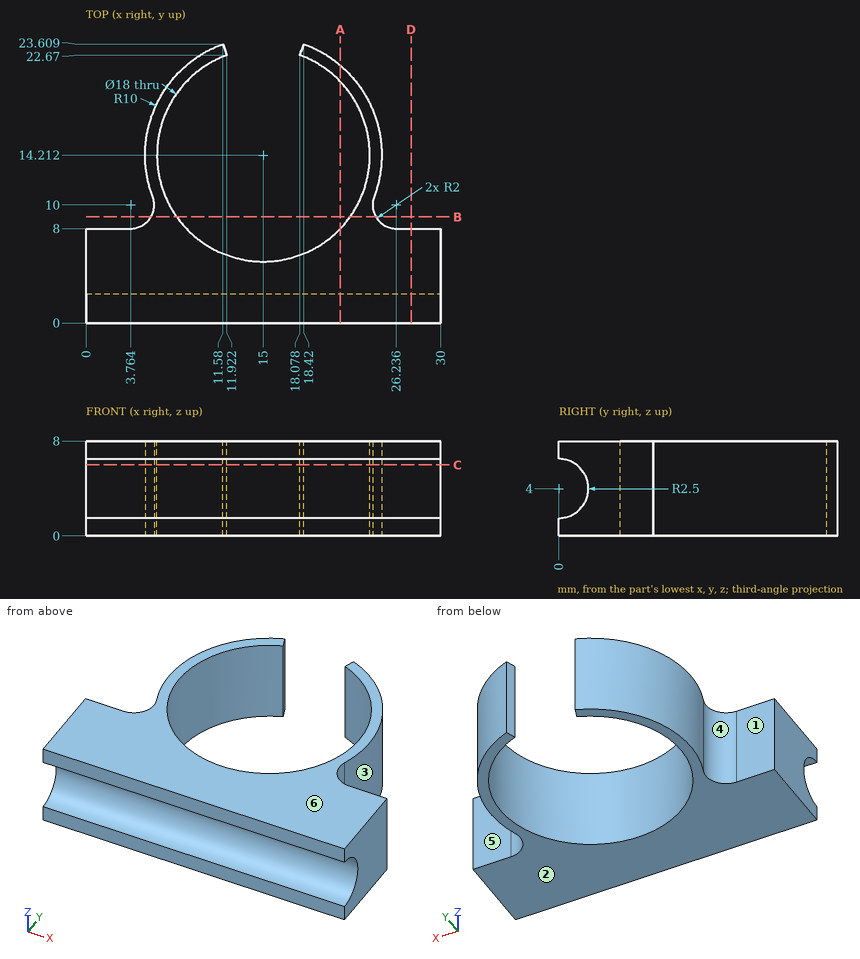
The drawing under review shows one solid part. Ordinate dimensions are in mm from its lowest x, y, z. A direction names the side the tool comes from. Round coordinates to 2 decimals unless told otherwise and drop trailing zeros. Loops run counter-clockwise (first coordinate to the right, second up) from the corner with the lowest first, then second, coordinate; pieces in that order, holes last.
Item 1: For the marked faces 1 and 2, list the 3-axis set-ups (+Z, -Z, +X, -X, +Y, -Y) from which the entire face can be reached by the end or side of a thin tool; tool diameter is ignored.
Determined:
face 1: +Z, -Z, -X, +Y
face 2: -Z, +X, -X, +Y, -Y
Item 2: Clearance check with flat-ended pins moving along their axes: pin 1 Ø4 at (y, z) = (16.5, 6.5) entering from +X; pin 2 Ø3 at (x, y) = (24.5, 16.5) entering from -Z; pin 3 Ø3 at (x, z) = (27.5, 3.5) entering from +Y; pin 4 Ø10 at (x, y) = (14, 12) entering from -Z. State where each tip first meets the part, or that it passes through.
Determined:
pin 1: stops at x = 25
pin 2: stops at z = 0
pin 3: stops at y = 8.01
pin 4: passes through
Item 3: For line 1 (X direction, y = 7.75, z = 3.25) (1 decimal); line 2 (X direction, y = 12, z = 3.25) (1 decimal); line 3 (Y direction, x = 10.75, z = 3.75) (1 decimal), list the stretches that pass through material, from the lowest coordinate up.
Determined:
line 1: x = 0 to 8.7, 21.3 to 30
line 2: x = 5.2 to 6.3, 23.7 to 24.8
line 3: y = 2.5 to 6.3, 22.1 to 23.3
Item 4: Take a section at D-D (x = 27.5). Write out the cut boundary in (y, z).
Determined:
outline: (0, 0) - (8, 0) - (8, 8) - (0, 8) - (0, 6.5) arc R2.5 cw to (0, 1.5) - close
Item 5: Take a section at B-B (y = 9). Write out the cut boundary in (x, z) (1 decimal).
Determined:
outline: (5.5, 0) - (7.7, 0) - (7.7, 8) - (5.5, 8) - close; (22.3, 0) - (24.5, 0) - (24.5, 8) - (22.3, 8) - close
Item 6: Take a section at A-A (x = 21.5). Write out the cut boundary in (y, z).
Determined:
outline: (0, 0) - (7.99, 0) - (7.99, 8) - (0, 8) - (0, 6.5) arc R2.5 cw to (0, 1.5) - close; (20.44, 0) - (21.81, 0) - (21.81, 8) - (20.44, 8) - close
Item 7: Mouldability with a two-part tool opening along Y and no side actions: class the marked faces 3, 4, 5 and 6 as released by +Y, released by -Y, zero draft, split by the parting line, or undercut.
Determined:
face 3: undercut
face 4: undercut
face 5: released by +Y
face 6: zero draft
Item 8: Take a section at C-C (z = 6). Write out the cut boundary in (x, y).
Determined:
outline: (0, 1.5) - (30, 1.5) - (30, 8) - (26.24, 8) arc R2 cw to (24.36, 10.7) arc R10 ccw to (18.42, 23.61) - (18.08, 22.67) arc R9 cw (long way) to (11.92, 22.67) - (11.58, 23.61) arc R10 ccw to (5.64, 10.7) arc R2 cw to (3.76, 8) - (0, 8) - close
